Solid Edge part; units mm, degrees
sketch "Sketch1" plane through (0, 0, 0) normal (0, -1, 0) x (1, 0, 0)
  line L0 (-45, -45) -> (-37, -45)
  line L1 (-37, -42) -> (-37, -45)
  line L2 (-19.6716, -22.5) -> (-37.3454, -40.1738)
  line L3 (-19.6716, -22.5) -> (19.6716, -22.5)
  line L4 (37.3454, -40.1738) -> (19.6716, -22.5)
  arc A0 (37, -42) -> (37.3454, -40.1738) centre (42, -42) cw
  line L5 (37, -42) -> (37, -45)
  line L6 (37, -45) -> (45, -45)
  line L7 (45, -45) -> (45, -37)
  line L8 (42, -37) -> (45, -37)
  line L9 (25.3284, -22.5) -> (40.1738, -37.3454)
  line L10 (25.3284, -22.5) -> (37.4174, -22.5)
  arc A1 (42, -25.5) -> (37.4174, -22.5) centre (42, -20.5) cw
  line L11 (42, -25.5) -> (45, -25.5)
  line L12 (45, -25.5) -> (45, -15.5)
  line L13 (42, -15.5) -> (45, -15.5)
  line L14 (37.4174, -18.5) -> (21.3284, -18.5)
  line L15 (2.8284, 0) -> (21.3284, -18.5)
  line L16 (21.3284, 18.5) -> (2.8284, 0)
  line L17 (21.3284, 18.5) -> (37.4174, 18.5)
  line L18 (42, 15.5) -> (45, 15.5)
  line L19 (45, 15.5) -> (45, 25.5)
  line L20 (42, 25.5) -> (45, 25.5)
  arc A2 (37.4174, 22.5) -> (42, 25.5) centre (42, 20.5) cw
  line L21 (37.4174, 22.5) -> (25.3284, 22.5)
  line L22 (40.1738, 37.3454) -> (25.3284, 22.5)
  line L23 (42, 37) -> (45, 37)
  line L24 (45, 37) -> (45, 45)
  line L25 (45, 45) -> (37, 45)
  line L26 (37, 42) -> (37, 45)
  arc A3 (37.3454, 40.1738) -> (37, 42) centre (42, 42) cw
  line L27 (19.6716, 22.5) -> (37.3454, 40.1738)
  line L28 (19.6716, 22.5) -> (-19.6716, 22.5)
  line L29 (-37.3454, 40.1738) -> (-19.6716, 22.5)
  line L30 (-37, 42) -> (-37, 45)
  line L31 (-37, 45) -> (-45, 45)
  line L32 (-45, 45) -> (-45, 37)
  line L33 (-42, 37) -> (-45, 37)
  arc A4 (-40.1738, 37.3454) -> (-42, 37) centre (-42, 42) cw
  line L34 (-25.3284, 22.5) -> (-40.1738, 37.3454)
  line L35 (-25.3284, 22.5) -> (-37.4174, 22.5)
  arc A5 (-42, 25.5) -> (-37.4174, 22.5) centre (-42, 20.5) cw
  line L36 (-42, 25.5) -> (-45, 25.5)
  line L37 (-45, 25.5) -> (-45, 15.5)
  line L38 (-42, 15.5) -> (-45, 15.5)
  line L39 (-37.4174, 18.5) -> (-21.3284, 18.5)
  line L40 (-2.8284, 0) -> (-21.3284, 18.5)
  line L41 (-21.3284, -18.5) -> (-2.8284, 0)
  line L42 (-21.3284, -18.5) -> (-37.4174, -18.5)
  arc A6 (-42, -15.5) -> (-37.4174, -18.5) centre (-42, -20.5) cw
  line L43 (-42, -15.5) -> (-45, -15.5)
  line L44 (-45, -15.5) -> (-45, -25.5)
  line L45 (-42, -25.5) -> (-45, -25.5)
  line L46 (-37.4174, -22.5) -> (-25.3284, -22.5)
  line L47 (-40.1738, -37.3454) -> (-25.3284, -22.5)
  arc A7 (-42, -37) -> (-40.1738, -37.3454) centre (-42, -42) cw
  line L48 (-42, -37) -> (-45, -37)
  line L49 (-45, -37) -> (-45, -45)
  arc A8 (-37, -42) -> (-37.3454, -40.1738) centre (-42, -42) ccw
  arc A9 (42, -37) -> (40.1738, -37.3454) centre (42, -42) ccw
  arc A10 (42, -15.5) -> (37.4174, -18.5) centre (42, -20.5) ccw
  arc A11 (37.4174, 18.5) -> (42, 15.5) centre (42, 20.5) ccw
  arc A12 (40.1738, 37.3454) -> (42, 37) centre (42, 42) ccw
  arc A13 (-37.3454, 40.1738) -> (-37, 42) centre (-42, 42) ccw
  arc A14 (-42, 15.5) -> (-37.4174, 18.5) centre (-42, 20.5) ccw
  arc A15 (-42, -25.5) -> (-37.4174, -22.5) centre (-42, -20.5) ccw
  circle A16 centre (-42, -42) radius 1.6
  circle A17 centre (42, -42) radius 1.6
  circle A18 centre (42, -20.5) radius 1.6
  circle A19 centre (-42, -20.5) radius 1.6
  circle A20 centre (-42, 20.5) radius 1.6
  circle A21 centre (-42, 42) radius 1.6
  circle A22 centre (42, 42) radius 1.6
  circle A23 centre (42, 20.5) radius 1.6
  line L50 (-15.6716, 18.5) -> (15.6716, 18.5)
  line L51 (0, 2.8284) -> (15.6716, 18.5)
  line L52 (-15.6716, 18.5) -> (0, 2.8284)
  line L53 (15.6716, -18.5) -> (-15.6716, -18.5)
  line L54 (0, -2.8284) -> (-15.6716, -18.5)
  line L55 (15.6716, -18.5) -> (0, -2.8284)
  dimension "D1" = 42
extrude "Protrusion1" add sketch "Sketch1" against normal blind 3
fillet "Round1" radius 1 20 edges at (-19.6716, 1.5, 22.5) (-25.3284, 1.5, 22.5) (19.6716, 1.5, 22.5) (25.3284, 1.5, 22.5) (21.3284, 1.5, 18.5) (15.6716, 1.5, 18.5) (-15.6716, 1.5, 18.5) (0, 1.5, 2.8284) (21.3284, 1.5, -18.5) (2.8284, 1.5, 0) (-2.8284, 1.5, 0) (19.6716, 1.5, -22.5) (-19.6716, 1.5, -22.5) (-15.6716, 1.5, -18.5) (0, 1.5, -2.8284) (15.6716, 1.5, -18.5) (25.3284, 1.5, -22.5) (-25.3284, 1.5, -22.5) (-21.3284, 1.5, -18.5) (-21.3284, 1.5, 18.5)
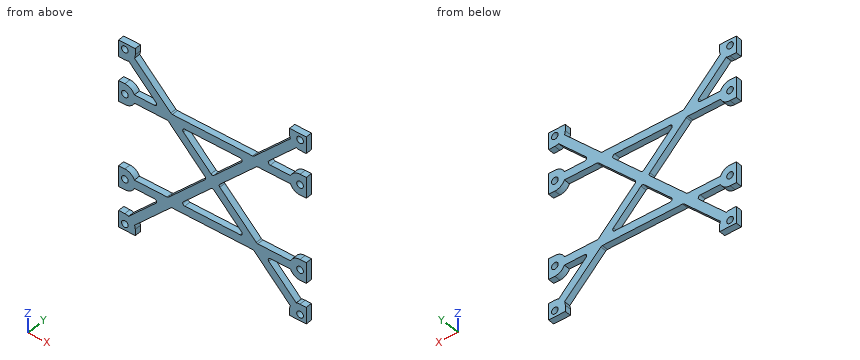
Design review of the part built by this model. Coordinates are the model's own, in mm. Give positions to 0.01 mm unless a question says otherwise; leave off trailing zeros. Loops run counter-clockwise (first coordinate to the right, second up) from the corner with the lowest first, then second, coordinate; pieces in that order, holes last. Notation, with made-up numbers: M 18.5,-15 L 41.5,-15 A24 cw 41.5,17 Z; hole C 81.5,66.5 d8. An arc over 180 degrees is marked long. Return JSON: item names as keys, results as strings. Group by question number.
Item 1: For probe 1 along Z at (x, y) = (-30.5, 1.15); probe 2 along Z at (x, y) = (-34.5, 1.85); probe 3 along X at (y, z) = (1.6, 23), list the stretches that pass through material, from the lowest coordinate up.
Item 2: Insertion check: pin 1 Ø1.9 at (x, z) = (42, 20.5) entering from -Y; pin 2 Ø0.9 at (x, y) = (-34, 2) entering from +Z. Each pin has a flat end and moves straight along its axis. Give the tip position at first contact, or say it passes through.
Item 3: We need section C-C (z = -39). Give the boundary of the cut face in (x, y).
Item 4: We need section D-D (x = 5). Give the boundary of the cut face in (y, z), and give its area (3 significant figures).
Item 5: We need section A-A (z = -20.5). Give the boundary of the cut face in (x, y).
Item 6: We need section B-B (x = -23). Give the boundary of the cut face in (y, z).
Output:
{
 "1": {"probe 1": "z = -33.33 to -27.67, -22.5 to -18.5, 18.5 to 22.5, 27.67 to 33.33", "probe 2": "z = -37.33 to -31.67, -22.5 to -18.5, 18.5 to 22.5, 31.67 to 37.33", "probe 3": "x = -45 to -37.67, -26.88 to -20.17, 20.17 to 26.88, 37.67 to 45"},
 "2": {"pin 1": "passes through", "pin 2": "stops at z = 37.28"},
 "3": {"outline": "M -45,0 L -36.17,0 L -36.17,3 L -45,3 Z; M 36.17,0 L 45,0 L 45,3 L 36.17,3 Z"},
 "4": {"outline": "M 0,-22.5 L 3,-22.5 L 3,-18.5 L 0,-18.5 Z; M 0,-7.83 L 3,-7.83 L 3,-2.17 L 0,-2.17 Z; M 0,2.17 L 3,2.17 L 3,7.83 L 0,7.83 Z; M 0,18.5 L 3,18.5 L 3,22.5 L 0,22.5 Z", "area": "57.9 mm^2"},
 "5": {"outline": "M -45,0 L -43.6,0 L -43.6,3 L -45,3 Z; M -40.4,0 L 40.4,0 L 40.4,3 L -40.4,3 Z; M 43.6,0 L 45,0 L 45,3 L 43.6,3 Z"},
 "6": {"outline": "M 0,-25.83 L 3,-25.83 L 3,-18.5 L 0,-18.5 Z; M 0,18.5 L 3,18.5 L 3,25.83 L 0,25.83 Z"}
}
